Part model, mm, in its own coordinate system. A direction names the side the tool comes from. Round coordinates to 2 decimals unless told otherwise and drop trailing zeros. One line per question, with ' | ' between items.
from build123d import *

# Parameters (mm, degrees)
SKETCH1_W           = 50
SKETCH1_H           = 50
BOSS_EXTRUDE1_DEPTH = 5
SKETCH2_W           = 50
SKETCH2_H           = 1.5
BOSS_EXTRUDE2_DEPTH = 10


with BuildPart() as part:
    # Sketch1 → Boss-Extrude1 (new body)
    with BuildSketch(Plane.XY):
        Rectangle(SKETCH1_W, SKETCH1_H)
    extrude(amount=BOSS_EXTRUDE1_DEPTH)

    # Sketch2 → Boss-Extrude2 (add)
    with BuildSketch(Plane.XY.offset(5)):
        with Locations((0, 24.25)):
            Rectangle(SKETCH2_W, SKETCH2_H)
        with Locations((0, 21.75)):
            Rectangle(SKETCH2_W, SKETCH2_H)
        with Locations((0, 19.25)):
            Rectangle(SKETCH2_W, SKETCH2_H)
        with Locations((0, 16.75)):
            Rectangle(SKETCH2_W, SKETCH2_H)
        with Locations((0, 14.25)):
            Rectangle(SKETCH2_W, SKETCH2_H)
        with Locations((0, 11.75)):
            Rectangle(SKETCH2_W, SKETCH2_H)
        with Locations((0, 9.25)):
            Rectangle(SKETCH2_W, SKETCH2_H)
        with Locations((0, 6.75)):
            Rectangle(SKETCH2_W, SKETCH2_H)
        with Locations((0, 4.25)):
            Rectangle(SKETCH2_W, SKETCH2_H)
        with Locations((0, 1.75)):
            Rectangle(SKETCH2_W, SKETCH2_H)
        with Locations((0, -0.75)):
            Rectangle(SKETCH2_W, SKETCH2_H)
        with Locations((0, -3.25)):
            Rectangle(SKETCH2_W, SKETCH2_H)
        with Locations((0, -5.75)):
            Rectangle(SKETCH2_W, SKETCH2_H)
        with Locations((0, -8.25)):
            Rectangle(SKETCH2_W, SKETCH2_H)
        with Locations((0, -10.75)):
            Rectangle(SKETCH2_W, SKETCH2_H)
        with Locations((0, -13.25)):
            Rectangle(SKETCH2_W, SKETCH2_H)
        with Locations((0, -15.75)):
            Rectangle(SKETCH2_W, SKETCH2_H)
        with Locations((0, -18.25)):
            Rectangle(SKETCH2_W, SKETCH2_H)
        with Locations((0, -20.75)):
            Rectangle(SKETCH2_W, SKETCH2_H)
        with Locations((0, -23.25)):
            Rectangle(SKETCH2_W, SKETCH2_H)
    extrude(amount=BOSS_EXTRUDE2_DEPTH)


solid = part.part
1) Saw through at A-A (z = 8). Give the number of separate pieces and of enclosed holes in the cut face, plus the area to 3 significant figures.
The answers:
separate pieces: 20 | enclosed holes: 0 | area: 1,500 mm²
2) Two-plate mould, pull along Y, no slides. Class faces 1 (the face through (0, -14, 10)), 2 (the face through (0, -6, 15)), 3 (the face through (0, -25, 2)): released by +Y, released by -Y, zero draft, split by the parting line, or undercut.
The answers:
face 1: undercut | face 2: zero draft | face 3: released by -Y
3) Probe line 1 (Z direction, x = -10.5, y = 23). List the from-to ranges inside material, lowest first. Write a range as [from, to].
The answers:
line 1: z = [0, 5]
4) Which spindle directions (+Z, -Z, +X, -X, +Y, -Y) get a long thin tool onto all of the face, cutting with end or side? Do faces 4 (the face through (0, 13.5, 10)), 5 (the face through (0, -11, 15)). Say none if no direction does.
The answers:
face 4: +Z, +X, -X | face 5: +Z, +X, -X, +Y, -Y
5) Drop flat-ended pins along their axis: pin 1 (5 mm diameter, centred on x = -3, z = 8, fed in from -Y); pin 2 (1.1 mm diameter, centred on x = 8.5, y = 23, fed in from +Z). Give the stop position or say it passes through.
The answers:
pin 1: stops at y = -24 | pin 2: stops at z = 15
